Source: CAD feature listing. Evaluate the final solid. Frame: model axes, mm. A direction names the side the tool comes from. Give positions to 0.01 mm unless a question says otherwise; leave off trailing zeros. Order: outer loops, then holes, each group sorted by start corner. A loop starts at its lowest first (then second) coordinate and runs counter-clockwise, first axis right, second up.
```python
from build123d import *

# Parameters (mm, degrees)
F0_R     = 1.5
F0_R_2   = 2
F1_DEPTH = 5
F2_R     = 5
F3_SIZE2 = 2.49999
F3_SIZE  = 2.49999


# Not quite as in the source:
# - a fillet or chamfer is up to 0.001 mm smaller than in the source, because OpenCascade refuses the exact size


with BuildPart() as f1:
    # F0 (on Top) → F1 (new body)
    with BuildSketch(Plane.XY):
        with BuildLine():
            Line((57, 4), (0, 4))
            Line((0, 4), (0, -4))
            Line((0, -4), (57, -4))
            ThreePointArc((57, -4), (65, 0), (57, 4))
        make_face()
        with Locations((40, 0)):
            Circle(F0_R, mode=Mode.SUBTRACT)
        with Locations((60, 0)):
            Circle(F0_R_2, mode=Mode.SUBTRACT)
        with BuildLine():
            Line((0, 4), (-57, 4))
            ThreePointArc((-57, 4), (-65, 0), (-57, -4))
            Line((-57, -4), (0, -4))
            Line((0, -4), (0, 4))
        make_face()
        with Locations((-60, 0)):
            Circle(F0_R_2, mode=Mode.SUBTRACT)
        with Locations((-40, 0)):
            Circle(F0_R, mode=Mode.SUBTRACT)
    extrude(amount=F1_DEPTH)

    # F2
    f2_edges = [f1.edges().sort_by_distance(p)[0] for p in [
        (-57, 4, 2.5),
        (-57, -4, 2.5),
        (57, -4, 2.5),
        (57, 4, 2.5),
    ]]
    fillet(f2_edges, radius=F2_R)

    # F3 (size 2.5 and 2.5 in the source; OpenCascade refuses exactly that, so slightly less here)
    f3_edges = [f1.edges().sort_by_distance(p)[0] for p in [
        (38.5, 0, 5),
        (-41.5, 0, 5),
        (-62, 0, 0),
        (58, 0, 0),
    ]]
    chamfer(f3_edges, length=F3_SIZE, length2=F3_SIZE2)


solid = f1.part
```
1) Section query C-C, the plane z = 4.2. Return the cut outline in (x, y).
Report:
outline: (-57.82, -4.5) arc R5 cw to (-55.64, -4) - (55.64, -4) arc R5 cw to (57.82, -4.5) arc R5 ccw (long way) to (57.82, 4.5) arc R5 cw to (55.64, 4) - (-55.64, 4) arc R5 cw to (-57.82, 4.5) arc R5 ccw (long way) to start; hole circle Ø4 at (-60, 0); hole circle Ø6.4 at (-40, 0); hole circle Ø6.4 at (40, 0); hole circle Ø4 at (60, 0)
2) Reachability of faces 1 (the flat face through (1, 4, 2)), 2 (the cylindrical face through (-58.153, -0.766, 3.732)) from +Z, -Z, +X, -X, +Y, -Y: full face, straight path, thin tool, end or side. Return the list, or none.
Report:
face 1: +Z, -Z, +Y
face 2: +Z, -Z
3) Draft query along Y for faces 3 (the flat face through (-1, -4, 2)), 4 (the flat face through (-1, 0, 0)), 5 (the cylindrical face through (-41.5, 0.07, 1.23)). Return one class per face: +Y half, -Y half, draft (parallel to the pull), parting line (faces both ways), or undercut.
Report:
face 3: -Y half
face 4: draft
face 5: undercut
4) Pin query (flat end, axial travel): pin 1 (3 mm diameter, centred on x = 60, y = 0, fed in from -Z); pin 2 (1.5 mm diameter, centred on x = -5.5, z = 1.5, fed in from +Y); pin 3 (2.5 mm diameter, centred on x = -2, z = 3, fed in from -Y); pin 4 (5 mm diameter, centred on x = -40, y = 0, fed in from +Z). Return the tip coordinate at first contact, or that it passes through.
Report:
pin 1: passes through
pin 2: stops at y = 4
pin 3: stops at y = -4
pin 4: stops at z = 3.5
5) Section query B-B, the plane x = -60. Return the cut outline in (y, z).
Report:
outline: (-5, 0) - (-4.5, 0) - (-2, 2.5) - (-2, 5) - (-5, 5) - close; (2, 2.5) - (4.5, 0) - (5, 0) - (5, 5) - (2, 5) - close
6) Section query A-A, the plane y = 0. Return the cut outline in (x, z), and give its area (3 significant figures).
Report:
outline: (-65, 0) - (-64.5, 0) - (-62, 2.5) - (-62, 5) - (-65, 5) - close; (-58, 2.5) - (-55.5, 0) - (-41.5, 0) - (-41.5, 2.5) - (-44, 5) - (-58, 5) - close; (-38.5, 0) - (38.5, 0) - (38.5, 2.5) - (36, 5) - (-36, 5) - (-38.5, 2.5) - close; (41.5, 0) - (55.5, 0) - (58, 2.5) - (58, 5) - (44, 5) - (41.5, 2.5) - close; (62, 2.5) - (64.5, 0) - (65, 0) - (65, 5) - (62, 5) - close
area: 555 mm2
7) Material intervals for L1, parallel to Y at x = -40, z = 2; L2, parallel to X at y = -1, z = 2.4; L3, parallel to Y at x = -60, z = 3.5, sorted ascending.
Report:
L1: y = -4 to -1.5, 1.5 to 4
L2: x = -64.9 to -61.85, -58.15 to -41.12, -38.88 to 38.88, 41.12 to 58.15, 61.85 to 64.9
L3: y = -5 to -2, 2 to 5
